```python
from build123d import *

# Parameters (mm, degrees)
SKETCH_1_W          = 10
SKETCH_1_H          = 10
EXTRUDE_1_DEPTH     = 10
SKETCH_2_R          = 2.5
EXTRUDE_2_DEPTH     = 5
SKETCH_3_R          = 1
EXTRUDE_3_DEPTH     = 5
CUT_EXTRUDE_START   = -30
SKETCH_4_R          = 2.5
CUT_EXTRUDE_1_DEPTH = 30
SKETCH_5_R          = 1
CUT_EXTRUDE_2_DEPTH = 30
SKETCH_9_W          = 10
SKETCH_9_H          = 10
EXTRUDE_5_DEPTH     = 10
SKETCH_10_R         = 2
CUT_EXTRUDE_4_DEPTH = 20


with BuildPart() as part:
    # 草图1 → 凸台-拉伸1 (new body)
    with BuildSketch(Plane.XY):
        Rectangle(SKETCH_1_W, SKETCH_1_H)
    extrude(amount=EXTRUDE_1_DEPTH)

    # 草图2 → 凸台-拉伸2 (add)
    with BuildSketch(Plane.XY.offset(10)):
        Circle(SKETCH_2_R)
    extrude(amount=EXTRUDE_2_DEPTH)

    # 草图3 → 凸台-拉伸3 (add)
    with BuildSketch(Plane(origin=(5, 0, 0), x_dir=(0, 0, -1), z_dir=(1, 0, 0))):
        with Locations(Location((-5, 0, 0), (0, 0, 270))):
            Circle(SKETCH_3_R)
    extrude(amount=EXTRUDE_3_DEPTH)

    # 草图4 → 切除-拉伸1 (cut)
    with BuildSketch(Plane.XY.offset(15).offset(CUT_EXTRUDE_START)):
        with Locations(Location((0, 0, 0), (0, 0, 180))):
            Circle(SKETCH_4_R)
    extrude(amount=CUT_EXTRUDE_1_DEPTH, mode=Mode.SUBTRACT)

    # 草图5 → 切除-拉伸2 (cut)
    with BuildSketch(Plane(origin=(10, 0, 0), x_dir=(0, 0, -1), z_dir=(1, 0, 0)).offset(CUT_EXTRUDE_START)):
        with Locations((-5, 0)):
            Circle(SKETCH_5_R)
    extrude(amount=CUT_EXTRUDE_2_DEPTH, mode=Mode.SUBTRACT)

    # 草图9 → 凸台-拉伸5 (add)
    with BuildSketch(Plane(origin=(0, 0, 0), x_dir=(-1, 0, 0), z_dir=(0, 0, -1))):
        Rectangle(SKETCH_9_W, SKETCH_9_H)
    extrude(amount=EXTRUDE_5_DEPTH)

    # 草图10 → 切除-拉伸4 (cut)
    with BuildSketch(Plane(origin=(0, 0, -10), x_dir=(-1, 0, 0), z_dir=(0, 0, -1))):
        Circle(SKETCH_10_R)
    extrude(amount=-CUT_EXTRUDE_4_DEPTH, mode=Mode.SUBTRACT)


solid = part.part
```
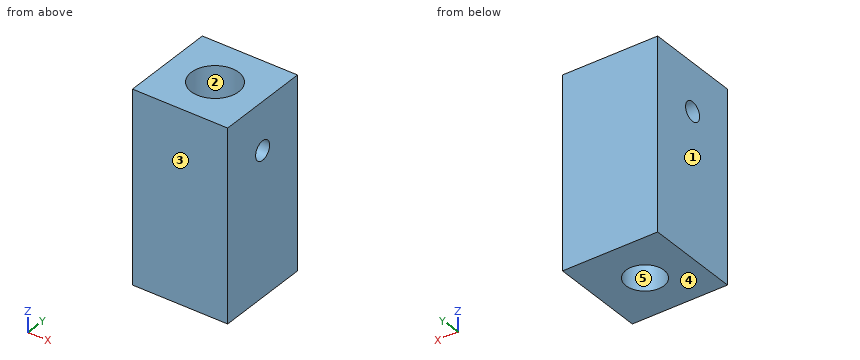
Check sheet for the modelled part. Datum: model origin and axes. Units: mm. Face numbers are marked on the shaded views. A direction names the side the tool comes from. Give positions to 0.01 mm unless a question says otherwise; leave off trailing zeros. Write each loop counter-clockwise with the first axis right and the second up, starting at its lowest first coordinate (ties: lowest second). Pieces come first, ordered by that corner, then holes.
Item 1: Access from +Z, -Z, +X, -X, +Y, -Y to the whole of each face (thin tool, end or side, straight path). Record for the marked faces 1 and 2.
Item 2: Scan lines: L1, parallel to Y at x = 0, z = -7; L2, parallel to X at y = -1, z = 7; L3, parallel to Y at x = 0, z = 4.75. Record each from-to range of solid material in increasing order.
Item 3: Cross-section at D-D (z = 1.25). Enter the section's corners in (x, y).
Item 4: Cross-section at C-C (y = 0). Enter the section's corners in (x, z), and give its area (3 significant figures).
Item 5: Cross-section at B-B (z = 5). Enter the section's corners in (x, y), and give its area (3 significant figures).
Item 6: Draft check along Y on the marked faces 3, 4 and 5. Enter one of: released by +Y, released by -Y, zero draft, split by the parting line, or undercut.
Item 7: Cross-section at A-A (x = 0). Enter the section's corners in (y, z).
Item 8: Gauge pin test, flat ends, axial feed: pin 1 (1.2 mm diameter, centred on y = 0, z = 5, fed in from -X); pin 2 (3 mm diameter, centred on x = 0.5, y = -0.5, fed in from -Z); pin 3 (2.5 mm diameter, centred on x = -0.5, y = -1, fed in from +Z). Record the tip position at first contact, or that the pin passes through.
Report:
1. face 1: +Z, -Z, -X, +Y, -Y
1. face 2: +Z
2. L1: y = -5 to -2, 2 to 5
2. L2: x = -5 to -2.29, 2.29 to 5
2. L3: y = -5 to -2.5, 2.5 to 5
3. outline: (-5, -5) - (5, -5) - (5, 5) - (-5, 5) - close; hole circle Ø5 at (0, 0)
4. outline: (-5, -10) - (-2, -10) - (-2, 0) - (-2.5, 0) - (-2.5, 4) - (-5, 4) - close; (-5, 6) - (-2.5, 6) - (-2.5, 10) - (-5, 10) - close; (2, -10) - (5, -10) - (5, 4) - (2.5, 4) - (2.5, 0) - (2, 0) - close; (2.5, 6) - (5, 6) - (5, 10) - (2.5, 10) - close
4. area: 100 mm2
5. outline: (-5, -5) - (5, -5) - (5, -1) - (2.29, -1) arc R2.5 cw to (-2.29, -1) - (-5, -1) - close; (-5, 1) - (-2.29, 1) arc R2.5 cw to (2.29, 1) - (5, 1) - (5, 5) - (-5, 5) - close
5. area: 70.1 mm2
6. face 3: released by -Y
6. face 4: zero draft
6. face 5: undercut
7. outline: (-5, -10) - (-2, -10) - (-2, 0) - (-2.5, 0) - (-2.5, 10) - (-5, 10) - close; (2, -10) - (5, -10) - (5, 10) - (2.5, 10) - (2.5, 0) - (2, 0) - close
8. pin 1: passes through
8. pin 2: stops at z = -10
8. pin 3: stops at z = 0
